```python
from build123d import *

# Parameters (mm, degrees)
BOSS_EXTRUDE1_DEPTH      = 1368.425
BOSS_EXTRUDE1_DEPTH_BACK = 1368.425
CUT_EXTRUDE1_DEPTH       = 48.625
CUT_EXTRUDE1_DEPTH_BACK  = 4.175


with BuildPart() as part:
    # Sketch4 → Boss-Extrude1 (new body, two sides)
    with BuildSketch(Plane.XY) as boss_extrude1_sk:
        with BuildLine():
            Line((-22.225, -18.838333333), (-22.225, 25.4))
            Line((-22.225, 25.4), (-25.4, 25.4))
            Line((-25.4, 25.4), (-25.4, -25.4))
            Line((-25.4, -25.4), (25.4, -25.4))
            Line((25.4, -25.4), (25.4, -22.225))
            Line((25.4, -22.225), (-18.838333333, -22.225))
            ThreePointArc((-18.838333333, -22.225), (-21.233068299, -21.233068299), (-22.225, -18.838333333))
        make_face()
    extrude(amount=BOSS_EXTRUDE1_DEPTH)
    extrude(boss_extrude1_sk.sketch, amount=-BOSS_EXTRUDE1_DEPTH_BACK)

    # Sketch5 → Cut-Extrude1 (cut, two sides)
    with BuildSketch(Plane(origin=(0, -22.225, 0), x_dir=(1, 0, 0), z_dir=(0, 1, 0))) as cut_extrude1_sk:
        Polygon((-25.4, 1368.425), (25.4, 1317.625), (25.4, 1368.425), align=None)
        Polygon((25.4, -1368.425), (-25.4, -1368.425), (25.4, -1317.625), align=None)
    extrude(amount=CUT_EXTRUDE1_DEPTH, mode=Mode.SUBTRACT)
    extrude(cut_extrude1_sk.sketch, amount=-CUT_EXTRUDE1_DEPTH_BACK, mode=Mode.SUBTRACT)


solid = part.part
```
Model file for the job. Use its own axes, mm. A direction names the side the tool comes from. Coordinates: 2 decimals unless noted, no trailing zeros. Write each loop counter-clockwise with the first axis right and the second up, starting at its lowest first coordinate (ties: lowest second). Pieces come first, ordered by that corner, then holes. Notation, with made-up numbers: (-23.5, 33.5) - (6.5, 33.5) arc R16 cw to (6.5, 54.5) - close; hole circle Ø5 at (22, 84.5). An arc over 180 degrees is marked (long way). One line per item, written item: value. Start each with the question number.
1. Flat gauge pins, fed straight in: pin 1 (13.5 mm diameter, centred on y = 11, z = 95.5, fed in from +X) (3 decimals); pin 2 (8 mm diameter, centred on x = -17.5, y = -8.5, fed in from -Z); pin 3 (8 mm diameter, centred on x = 12.5, y = -19.5, fed in from -Z). Where does each tip first touch, or does it go through?
2. Slice it at B-B (x = 5). Write the cut outline in (y, z) (3 decimals).
3. Slice it at A-A (z = 642). Write the cut outline in (x, y) (3 decimals).
4. Tool access for faces 1 (the flat face through (4, -22.225, 19)), 2 (the flat face through (-25.4, 0, 19)): list every direction of +Z, -Z, +X, -X, +Y, -Y with a clear straight run to the whole face (end or side of a thin tool).
5. Probe line 1 (Y direction, x = -5.5, z = 839.5) (3 decimals); line 2 (X direction, y = -20.5, z = -39.5). List the from-to ranges inside material, lowest first. Write a range as from..to.
6. Slice it at C-C (y = 4). Write the cut outline in (x, z) (3 decimals), plus the area to 3 significant figures.
Answers below:
1. pin 1: stops at x = -22.225
1. pin 2: passes through
1. pin 3: stops at z = -1333.45
2. outline: (-25.4, -1338.025) - (-22.225, -1338.025) - (-22.225, 1338.025) - (-25.4, 1338.025) - close
3. outline: (-25.4, -25.4) - (25.4, -25.4) - (25.4, -22.225) - (-18.838, -22.225) arc R3.387 cw to (-22.225, -18.838) - (-22.225, 25.4) - (-25.4, 25.4) - close
4. face 1: +Z, -Z, +X, +Y
4. face 2: +Z, -Z, -X, +Y, -Y
5. line 1: y = -25.4..-22.225
5. line 2: x = -25.4..-21.79
6. outline: (-25.4, -1368.425) - (-22.225, -1365.25) - (-22.225, 1365.25) - (-25.4, 1368.425) - close
6. area: 8,680 mm^2
